Read the model definition and answer for the solid it produces. Units are mm, in the model's axes. Coordinates: 2 decimals unless noted, no trailing zeros. Write each loop counter-clockwise with the first axis right and the second up, starting at its lowest first coordinate (ties: lowest second). Pieces come first, ordered by that corner, then holes. Notation, with made-up numbers: (1.25, -10) -> (50.25, -10) arc R22 ccw to (50.25, 3) -> close; hole circle Ø10 at (-33, 68.5). An arc over 180 degrees is marked (long way). Return JSON: item names as keys, results as strings.
from build123d import *

# Parameters (mm, degrees)
F0_R     = 1
F0_R_2   = 5.5
F1_DEPTH = 3.175


with BuildPart() as f1:
    # F0 (on Top) → F1 (new body)
    with BuildSketch(Plane.XY):
        with BuildLine():
            Line((42.5, 0), (49, 0))
            ThreePointArc((49, 0), (0, 49), (-49, 0))
            Line((-49, 0), (-42.5, 0))
            ThreePointArc((-42.5, 0), (-35, 7.5), (-27.5, 0))
            Line((-27.5, 0), (0, 0))
            Line((0, 0), (27.5, 0))
            ThreePointArc((27.5, 0), (35, 7.5), (42.5, 0))
        make_face()
        Polygon((25.5, 6), (0, 6), (-25.5, 6), (-25.5, 18), (0, 18), (25.5, 18), align=None, mode=Mode.SUBTRACT)
        with Locations((-31.8198051534, 31.8198051534)):
            Circle(F0_R, mode=Mode.SUBTRACT)
        with BuildLine():
            ThreePointArc((5.5, 35), (3.8890872965, 31.1109127035), (0, 29.5))
            ThreePointArc((0, 29.5), (-3.8890872965, 38.8890872965), (5.5, 35))
        make_face(mode=Mode.SUBTRACT)
        with Locations((31.8198051534, 31.8198051534)):
            Circle(F0_R, mode=Mode.SUBTRACT)
        with BuildLine():
            ThreePointArc((-49, 0), (0, -49), (49, 0))
            Line((49, 0), (42.5, 0))
            ThreePointArc((42.5, 0), (35, -7.5), (27.5, 0))
            Line((27.5, 0), (0, 0))
            Line((0, 0), (-27.5, 0))
            ThreePointArc((-27.5, 0), (-35, -7.5), (-42.5, 0))
            Line((-42.5, 0), (-49, 0))
        make_face()
        with BuildLine():
            ThreePointArc((-30.8198051534, -31.8198051534), (-32.7436846859, -32.2024885858), (-31.1126983722, -31.1126983722))
            ThreePointArc((-31.1126983722, -31.1126983722), (-30.8959256209, -31.437121721), (-30.8198051534, -31.8198051534))
        make_face(mode=Mode.SUBTRACT)
        with BuildLine():
            ThreePointArc((-3.25, -35), (-4.9571067812, -35.7071067812), (-4.25, -34))
            ThreePointArc((-4.25, -34), (-3.5428932188, -34.2928932188), (-3.25, -35))
        make_face(mode=Mode.SUBTRACT)
        with BuildLine():
            ThreePointArc((-4.25, -31), (-5.25, -30), (-4.25, -29))
            ThreePointArc((-4.25, -29), (-3.5428932188, -29.2928932188), (-3.25, -30))
            ThreePointArc((-3.25, -30), (-3.5428932188, -30.7071067812), (-4.25, -31))
        make_face(mode=Mode.SUBTRACT)
        with BuildLine():
            ThreePointArc((-4.25, -26), (-5.25, -25), (-4.25, -24))
            ThreePointArc((-4.25, -24), (-3.5428932188, -24.2928932188), (-3.25, -25))
            ThreePointArc((-3.25, -25), (-3.5428932188, -25.7071067812), (-4.25, -26))
        make_face(mode=Mode.SUBTRACT)
        with Locations((-30.3108891325, -17.5)):
            Circle(F0_R_2, mode=Mode.SUBTRACT)
        with BuildLine():
            ThreePointArc((-4.25, -21), (-5.25, -20), (-4.25, -19))
            ThreePointArc((-4.25, -19), (-3.5428932188, -19.2928932188), (-3.25, -20))
            ThreePointArc((-3.25, -20), (-3.5428932188, -20.7071067812), (-4.25, -21))
        make_face(mode=Mode.SUBTRACT)
        with BuildLine():
            ThreePointArc((-4.25, -16), (-5.25, -15), (-4.25, -14))
            ThreePointArc((-4.25, -14), (-3.5428932188, -14.2928932188), (-3.25, -15))
            ThreePointArc((-3.25, -15), (-3.5428932188, -15.7071067812), (-4.25, -16))
        make_face(mode=Mode.SUBTRACT)
        with BuildLine():
            ThreePointArc((-4.25, -11), (-4.9571067812, -9.2928932188), (-3.25, -10))
            ThreePointArc((-3.25, -10), (-3.5428932188, -10.7071067812), (-4.25, -11))
        make_face(mode=Mode.SUBTRACT)
        with BuildLine():
            ThreePointArc((5.25, -35), (3.5428932188, -35.7071067812), (4.25, -34))
            ThreePointArc((4.25, -34), (4.9571067812, -34.2928932188), (5.25, -35))
        make_face(mode=Mode.SUBTRACT)
        with BuildLine():
            ThreePointArc((4.25, -31), (3.25, -30), (4.25, -29))
            ThreePointArc((4.25, -29), (4.9571067812, -29.2928932188), (5.25, -30))
            ThreePointArc((5.25, -30), (4.9571067812, -30.7071067812), (4.25, -31))
        make_face(mode=Mode.SUBTRACT)
        with BuildLine():
            ThreePointArc((4.25, -26), (3.25, -25), (4.25, -24))
            ThreePointArc((4.25, -24), (4.9571067812, -24.2928932188), (5.25, -25))
            ThreePointArc((5.25, -25), (4.9571067812, -25.7071067812), (4.25, -26))
        make_face(mode=Mode.SUBTRACT)
        with Locations((31.8198051534, -31.8198051534)):
            Circle(F0_R, mode=Mode.SUBTRACT)
        with BuildLine():
            ThreePointArc((4.25, -21), (3.25, -20), (4.25, -19))
            ThreePointArc((4.25, -19), (4.9571067812, -19.2928932188), (5.25, -20))
            ThreePointArc((5.25, -20), (4.9571067812, -20.7071067812), (4.25, -21))
        make_face(mode=Mode.SUBTRACT)
        with BuildLine():
            ThreePointArc((4.25, -16), (3.25, -15), (4.25, -14))
            ThreePointArc((4.25, -14), (4.9571067812, -14.2928932188), (5.25, -15))
            ThreePointArc((5.25, -15), (4.9571067812, -15.7071067812), (4.25, -16))
        make_face(mode=Mode.SUBTRACT)
        with BuildLine():
            ThreePointArc((4.25, -11), (3.5428932188, -10.7071067812), (3.25, -10))
            ThreePointArc((3.25, -10), (4.25, -9), (5.25, -10))
            ThreePointArc((5.25, -10), (4.9571067812, -10.7071067812), (4.25, -11))
        make_face(mode=Mode.SUBTRACT)
        with Locations((30.3108891325, -17.5)):
            Circle(F0_R_2, mode=Mode.SUBTRACT)
        Polygon((-25.5, 6), (0, 6), (0, 12), (0, 18), (-25.5, 18), align=None)
        Polygon((0, 12), (0, 6), (25.5, 6), (25.5, 18), (0, 18), align=None)
        with BuildLine():
            Line((-37.38, 0), (-42.5, 0))
            ThreePointArc((-42.5, 0), (-35, -7.5), (-27.5, 0))
            Line((-27.5, 0), (-32.62, 0))
            ThreePointArc((-32.62, 0), (-35, -2.38), (-37.38, 0))
        make_face()
        with BuildLine():
            ThreePointArc((-27.5, 0), (-35, 7.5), (-42.5, 0))
            Line((-42.5, 0), (-37.38, 0))
            ThreePointArc((-37.38, 0), (-35, 2.38), (-32.62, 0))
            Line((-32.62, 0), (-27.5, 0))
        make_face()
        with BuildLine():
            Line((37.38, 0), (42.5, 0))
            ThreePointArc((42.5, 0), (35, 7.5), (27.5, 0))
            Line((27.5, 0), (32.62, 0))
            ThreePointArc((32.62, 0), (35, 2.38), (37.38, 0))
        make_face()
        with BuildLine():
            ThreePointArc((27.5, 0), (35, -7.5), (42.5, 0))
            Line((42.5, 0), (37.38, 0))
            ThreePointArc((37.38, 0), (35, -2.38), (32.62, 0))
            Line((32.62, 0), (27.5, 0))
        make_face()
    extrude(amount=F1_DEPTH)


solid = f1.part
1. Consider L1, parallel to X at y = 2, z = 0.5; L2, parallel to X at y = 32, z = 0.9; L3, parallel to Y at x = 31.5, z = 2.4. Determine where each line is inside the solid, lowest interval first.
Taken from the geometry:
{"L1": "x = -48.96 to -36.29, -33.71 to 33.71, 36.29 to 48.96", "L2": "x = -37.11 to -32.8, -30.84 to -4.61, 4.61 to 30.84, 32.8 to 37.11", "L3": "y = -37.53 to -32.77, -30.87 to -22.87, -12.13 to 30.87, 32.77 to 37.53"}
2. Flat-ended cylindrical pins translate along their axes: pin 1 Ø14.5 at (x, y) = (-30.31, -17.5) entering from +Z (3 decimals); pin 2 Ø1 at (y, z) = (35, 0.5) entering from -X; pin 3 Ø1 at (x, z) = (-3, 2.5) entering from -Y; pin 4 Ø1 at (x, z) = (-1, 1.5) entering from -Y. Find the tip coordinate at first contact, or state that the pin passes through.
Taken from the geometry:
{"pin 1": "stops at z = 3.175", "pin 2": "stops at x = -34.8", "pin 3": "stops at y = -48.94", "pin 4": "stops at y = -49"}
3. The part is cut by section C-C (x = -23). Determine the outline of the cut face in (y, z) (3 decimals), then the cut area to 3 significant figures.
Taken from the geometry:
{"outline": "(-43.267, 0) -> (43.267, 0) -> (43.267, 3.175) -> (-43.267, 3.175) -> close", "area": "275 mm2"}
4. The part is cut by section B-B (y = -42). Determine the outline of the cut face in (x, z) (3 decimals), then the cut area to 3 significant figures.
Taken from the geometry:
{"outline": "(-25.239, 0) -> (25.239, 0) -> (25.239, 3.175) -> (-25.239, 3.175) -> close", "area": "160 mm2"}
5. For a pull along X with two mould halves and no side action, classify faces 1 (the face through (32.622, -0.105, 1.565)), 2 (the face through (-1, 1, 3.175)), 3 (the face through (-32.622, 0.105, 1.565)), 4 (the face through (-26.34, -41.32, 1.57)) as +X half, -X half, draft (parallel to the pull), parting line (faces both ways), or undercut.
Taken from the geometry:
{"face 1": "undercut", "face 2": "draft", "face 3": "undercut", "face 4": "parting line"}
6. The part is cut by section A-A (x = -34). Determine the outline of the cut face in (y, z) (3 decimals), then the cut area to 3 significant figures.
Taken from the geometry:
{"outline": "(-35.285, 0) -> (-21.579, 0) -> (-21.579, 3.175) -> (-35.285, 3.175) -> close; (-13.421, 0) -> (-2.16, 0) -> (-2.16, 3.175) -> (-13.421, 3.175) -> close; (2.16, 0) -> (35.285, 0) -> (35.285, 3.175) -> (2.16, 3.175) -> close", "area": "184 mm2"}
7. The part is cut by section D-D (z = 2.15). Count the separate pieces of the cut face and the enclosed holes in it, then the cut area to 3 significant figures.
Taken from the geometry:
{"separate pieces": "1", "enclosed holes": "21", "area": "7,170 mm2"}
